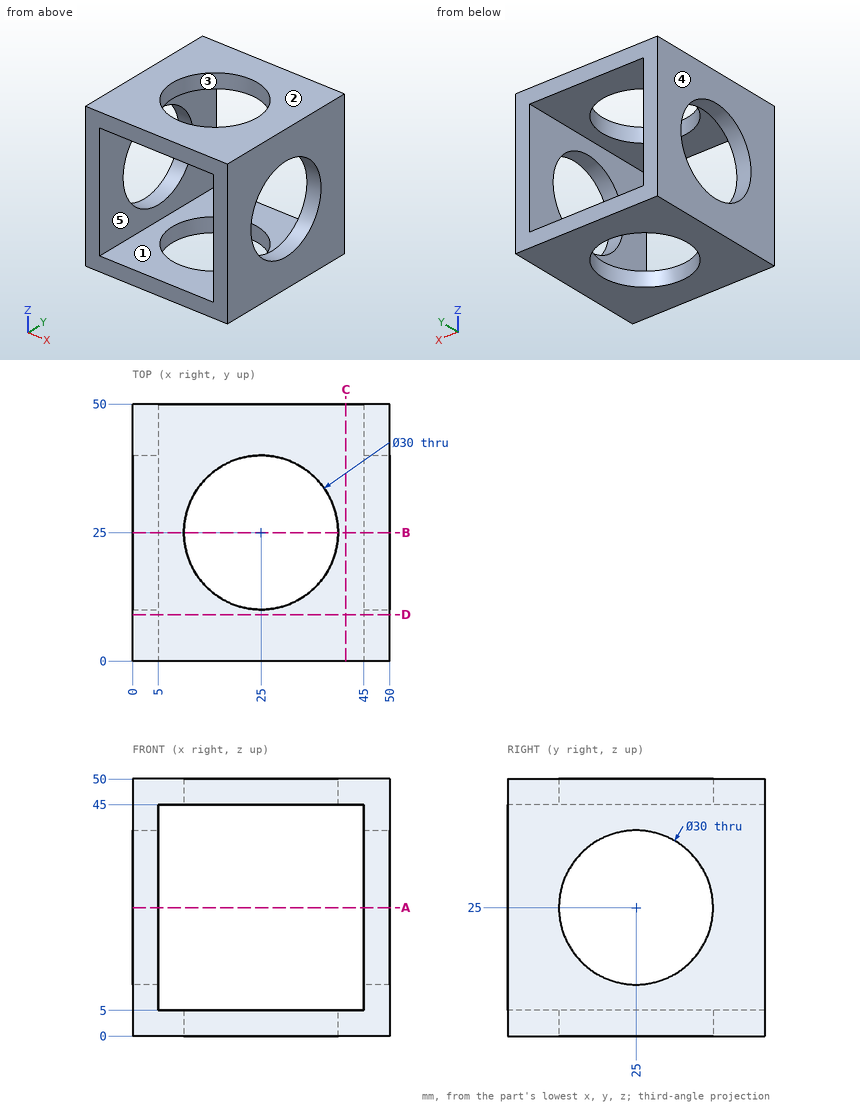
Study the drawing (mm; zero at the part's minimum x, y, z) and answer. A direction names the side the tool comes from. Give positions to 0.01 mm unless a question says otherwise; leave off trailing zeros. Loops run counter-clockwise (first coordinate to the right, second up) from the corner with the lowest first, then second, coordinate; pieces in that order, holes last. Notation, with made-up numbers: (-26, 59.25) - (7, 59.25) arc R8 ccw to (7, 72.25) - close; hole circle Ø9 at (53.5, -24.75). An arc over 180 degrees is marked (long way). Answer in a Markdown table with one row per item. Add a question column.
Q1. The part is cut by section B-B (y = 25). Determine the outline of the cut face in (x, z).
Q2. Each of these flat-tipped pins is pushed along its axis until it touches: P1, Ø8, axis at x = 24, y = 17, coming from the -Z side; P2, Ø20, axis at x = 33, y = 25.5, coming from the +Z side. Where does it stop, or does it pass through?
Q3. The part is cut by section D-D (y = 9). Determine the outline of the cut face in (x, z), and give its area (3 significant figures).
Q4. Determine the mould class of the marked faces 1, 2 and 3 for opening direction Z: released by +Z, released by -Z, zero draft, split by the parting line, or undercut.
Q5. The part is cut by section A-A (z = 25). Determine the outline of the cut face in (x, y).
Q6. The part is cut by section C-C (x = 41.5). Determine the outline of the cut face in (y, z).
Q7. A tool of negligible diameter and unlimited length cuts with its end or side. For the marked faces 4 and 5, from which of +Z, -Z, +X, -X, +Y, -Y can it reach the whole face along a straight path? Write none if from no direction.
Q8. Consider line 1 along X through (y, z) = (15, 12.5); line 2 along Y through (x, z) = (25, 48.05). Determine where each line is inside the solid, lowest interval first.
Solution:
| question | item | result |
|---|---|---|
| 1 | outline | (0, 0) - (10, 0) - (10, 5) - (5, 5) - (5, 10) - (0, 10) - close; (0, 40) - (5, 40) - (5, 45) - (10, 45) - (10, 50) - (0, 50) - close; (40, 0) - (50, 0) - (50, 10) - (45, 10) - (45, 5) - (40, 5) - close; (40, 45) - (45, 45) - (45, 40) - (50, 40) - (50, 50) - (40, 50) - close |
| 2 | P1 | passes through |
| 2 | P2 | stops at z = 50 |
| 3 | outline | (0, 0) - (50, 0) - (50, 50) - (0, 50) - close; hole (5, 5) - (45, 5) - (45, 45) - (5, 45) - close |
| 3 | area | 900 mm² |
| 4 | face 1 | undercut |
| 4 | face 2 | released by +Z |
| 4 | face 3 | zero draft |
| 5 | outline | (0, 0) - (5, 0) - (5, 10) - (0, 10) - close; (0, 40) - (5, 40) - (5, 50) - (0, 50) - close; (45, 0) - (50, 0) - (50, 10) - (45, 10) - close; (45, 40) - (50, 40) - (50, 50) - (45, 50) - close |
| 6 | outline | (0, 0) - (50, 0) - (50, 5) - (0, 5) - close; (0, 45) - (50, 45) - (50, 50) - (0, 50) - close |
| 7 | face 4 | +Z, -Z, -X, +Y, -Y |
| 7 | face 5 | +Y, -Y |
| 8 | line 1 | x = 0 to 5, 45 to 50 |
| 8 | line 2 | y = 0 to 10, 40 to 50 |
